The model under review builds one solid part; all positions refer to its coordinate system, in mm. A direction names the side the tool comes from. Round coordinates to 2 decimals unless told otherwise and drop trailing zeros. Order: outer loops, then holes, each group sorted by start corner. A loop starts at its lowest first (then second) coordinate and runs counter-clockwise, first axis right, second up. Notation, with made-up numbers: (-15, 65) -> (10, 65) arc R15 ccw to (10, 88) -> close; hole circle Ø3 at (56, -28). An arc over 180 degrees is marked (long way). Put each result on its own line as item: value. Start each with the question number.
from build123d import *

# Parameters (mm, degrees)
F1_DEPTH = 6
F2_DEPTH = 3
F3_START = 2
F3_DEPTH = 1
F4_SIZE  = 0.5
F5_DEPTH = 8
F6_START = -7.5
F6_DEPTH = 0.5
F7_R     = 0.49999


# Not quite as in the source:
# - a fillet or chamfer is up to 0.001 mm smaller than in the source, because OpenCascade refuses the exact size


with BuildPart() as f1:
    # F0 (on Front) → F1 (new body)
    with BuildSketch(Plane.XZ):
        with BuildLine():
            Line((2, 0), (4, 0))
            ThreePointArc((4, 0), (0, 4), (-4, 0))
            Line((-4, 0), (-2, 0))
            ThreePointArc((-2, 0), (-1.5491933385, 1.2649110641), (-0.4, 1.9595917942))
            Line((-0.4, 1.9595917942), (-0.4, 2))
            Line((-0.4, 2), (0, 2))
            Line((0, 2), (0.4, 2))
            Line((0.4, 2), (0.4, 1.9595917942))
            ThreePointArc((0.4, 1.9595917942), (1.5491933385, 1.2649110641), (2, 0))
        make_face()
        with BuildLine():
            Line((1.75, 0), (2, 0))
            ThreePointArc((2, 0), (1.5491933385, 1.2649110641), (0.4, 1.9595917942))
            Line((0.4, 1.9595917942), (0.4, 1.7036725037))
            ThreePointArc((0.4, 1.7036725037), (1.3715866724, 1.086853256), (1.75, 0))
        make_face()
        with BuildLine():
            ThreePointArc((-0.4, 1.9595917942), (-1.5491933385, 1.2649110641), (-2, 0))
            Line((-2, 0), (-1.75, 0))
            ThreePointArc((-1.75, 0), (-1.3715866724, 1.086853256), (-0.4, 1.7036725037))
            Line((-0.4, 1.7036725037), (-0.4, 1.9595917942))
        make_face()
        with BuildLine():
            Line((1.2, 0), (1.75, 0))
            ThreePointArc((1.75, 0), (1.3715866724, 1.086853256), (0.4, 1.7036725037))
            Line((0.4, 1.7036725037), (0.4, 1.1313708499))
            ThreePointArc((0.4, 1.1313708499), (0.9797958971, 0.692820323), (1.2, 0))
        make_face()
        with BuildLine():
            ThreePointArc((0, 2), (0.201017924, 1.989872306), (0.4, 1.9595917942))
            Line((0.4, 1.9595917942), (0.4, 2))
            Line((0.4, 2), (0, 2))
        make_face()
        with BuildLine():
            Line((0.4, 1.7036725037), (0.4, 1.9595917942))
            ThreePointArc((0.4, 1.9595917942), (0.201017924, 1.989872306), (0, 2))
            ThreePointArc((0, 2), (-0.201017924, 1.989872306), (-0.4, 1.9595917942))
            Line((-0.4, 1.9595917942), (-0.4, 1.7036725037))
            ThreePointArc((-0.4, 1.7036725037), (0, 1.75), (0.4, 1.7036725037))
        make_face()
        with BuildLine():
            ThreePointArc((-0.4, 1.7036725037), (-1.3715866724, 1.086853256), (-1.75, 0))
            Line((-1.75, 0), (-1.2, 0))
            ThreePointArc((-1.2, 0), (-0.9797958971, 0.692820323), (-0.4, 1.1313708499))
            Line((-0.4, 1.1313708499), (-0.4, 1.7036725037))
        make_face()
        with BuildLine():
            Line((-0.4, 2), (-0.4, 1.9595917942))
            ThreePointArc((-0.4, 1.9595917942), (-0.201017924, 1.989872306), (0, 2))
            Line((0, 2), (-0.4, 2))
        make_face()
        with BuildLine():
            Line((1, 0), (1.2, 0))
            ThreePointArc((1.2, 0), (0.9797958971, 0.692820323), (0.4, 1.1313708499))
            Line((0.4, 1.1313708499), (0.4, 0.916515139))
            ThreePointArc((0.4, 0.916515139), (0.8366600265, 0.5477225575), (1, 0))
        make_face()
        with BuildLine():
            Line((0.4, 1.1313708499), (0.4, 1.7036725037))
            ThreePointArc((0.4, 1.7036725037), (0, 1.75), (-0.4, 1.7036725037))
            Line((-0.4, 1.7036725037), (-0.4, 1.1313708499))
            ThreePointArc((-0.4, 1.1313708499), (0, 1.2), (0.4, 1.1313708499))
        make_face()
        with BuildLine():
            ThreePointArc((-0.4, 1.1313708499), (-0.9797958971, 0.692820323), (-1.2, 0))
            Line((-1.2, 0), (-1, 0))
            ThreePointArc((-1, 0), (-0.8366600265, 0.5477225575), (-0.4, 0.916515139))
            Line((-0.4, 0.916515139), (-0.4, 1.1313708499))
        make_face()
        with BuildLine():
            Line((0.4, 0), (1, 0))
            ThreePointArc((1, 0), (0.8366600265, 0.5477225575), (0.4, 0.916515139))
            Line((0.4, 0.916515139), (0.4, 0))
        make_face()
        with BuildLine():
            Line((0.4, 0.916515139), (0.4, 1.1313708499))
            ThreePointArc((0.4, 1.1313708499), (0, 1.2), (-0.4, 1.1313708499))
            Line((-0.4, 1.1313708499), (-0.4, 0.916515139))
            ThreePointArc((-0.4, 0.916515139), (0, 1), (0.4, 0.916515139))
        make_face()
        with BuildLine():
            ThreePointArc((-0.4, 0.916515139), (-0.8366600265, 0.5477225575), (-1, 0))
            Line((-1, 0), (-0.4, 0))
            Line((-0.4, 0), (-0.4, 0.916515139))
        make_face()
        with BuildLine():
            Line((-0.4, 0), (0.4, 0))
            Line((0.4, 0), (0.4, 0.916515139))
            ThreePointArc((0.4, 0.916515139), (0, 1), (-0.4, 0.916515139))
            Line((-0.4, 0.916515139), (-0.4, 0))
        make_face()
    extrude(amount=-F1_DEPTH)

    # F0 (on Front) → F2 (join)
    with BuildSketch(Plane.XZ):
        with BuildLine():
            ThreePointArc((-0.4, 1.7036725037), (-1.3715866724, 1.086853256), (-1.75, 0))
            Line((-1.75, 0), (-1.2, 0))
            ThreePointArc((-1.2, 0), (-0.9797958971, 0.692820323), (-0.4, 1.1313708499))
            Line((-0.4, 1.1313708499), (-0.4, 1.7036725037))
        make_face()
        with BuildLine():
            Line((1, 0), (1.2, 0))
            ThreePointArc((1.2, 0), (0.9797958971, 0.692820323), (0.4, 1.1313708499))
            Line((0.4, 1.1313708499), (0.4, 0.916515139))
            ThreePointArc((0.4, 0.916515139), (0.8366600265, 0.5477225575), (1, 0))
        make_face()
        with BuildLine():
            Line((1.2, 0), (1.75, 0))
            ThreePointArc((1.75, 0), (1.3715866724, 1.086853256), (0.4, 1.7036725037))
            Line((0.4, 1.7036725037), (0.4, 1.1313708499))
            ThreePointArc((0.4, 1.1313708499), (0.9797958971, 0.692820323), (1.2, 0))
        make_face()
        with BuildLine():
            ThreePointArc((-0.4, 1.1313708499), (-0.9797958971, 0.692820323), (-1.2, 0))
            Line((-1.2, 0), (-1, 0))
            ThreePointArc((-1, 0), (-0.8366600265, 0.5477225575), (-0.4, 0.916515139))
            Line((-0.4, 0.916515139), (-0.4, 1.1313708499))
        make_face()
    extrude(amount=F2_DEPTH)

    # F0 (on Front) → F3 (join)
    with BuildSketch(Plane.XZ.offset(F3_START)):
        with BuildLine():
            Line((1.75, 0), (2, 0))
            ThreePointArc((2, 0), (1.5491933385, 1.2649110641), (0.4, 1.9595917942))
            Line((0.4, 1.9595917942), (0.4, 1.7036725037))
            ThreePointArc((0.4, 1.7036725037), (1.3715866724, 1.086853256), (1.75, 0))
        make_face()
        with BuildLine():
            ThreePointArc((-0.4, 1.9595917942), (-1.5491933385, 1.2649110641), (-2, 0))
            Line((-2, 0), (-1.75, 0))
            ThreePointArc((-1.75, 0), (-1.3715866724, 1.086853256), (-0.4, 1.7036725037))
            Line((-0.4, 1.7036725037), (-0.4, 1.9595917942))
        make_face()
    extrude(amount=F3_DEPTH)

    # F4
    f4_edges = [f1.edges().sort_by_distance(p)[0] for p in [
        (0, 0, 4),
        (0, 6, 4),
    ]]
    chamfer(f4_edges, length=F4_SIZE)

    # F0 (on Front) → F5 (join)
    with BuildSketch(Plane.XZ):
        with BuildLine():
            Line((0.4, 0), (1, 0))
            ThreePointArc((1, 0), (0.8366600265, 0.5477225575), (0.4, 0.916515139))
            Line((0.4, 0.916515139), (0.4, 0))
        make_face()
        with BuildLine():
            ThreePointArc((-0.4, 0.916515139), (-0.8366600265, 0.5477225575), (-1, 0))
            Line((-1, 0), (-0.4, 0))
            Line((-0.4, 0), (-0.4, 0.916515139))
        make_face()
    extrude(amount=-F5_DEPTH)

    # F0 (on Front) → F6 (join)
    with BuildSketch(Plane.XZ.offset(F6_START)):
        with BuildLine():
            ThreePointArc((-0.4, 1.1313708499), (-0.9797958971, 0.692820323), (-1.2, 0))
            Line((-1.2, 0), (-1, 0))
            ThreePointArc((-1, 0), (-0.8366600265, 0.5477225575), (-0.4, 0.916515139))
            Line((-0.4, 0.916515139), (-0.4, 1.1313708499))
        make_face()
        with BuildLine():
            Line((1, 0), (1.2, 0))
            ThreePointArc((1.2, 0), (0.9797958971, 0.692820323), (0.4, 1.1313708499))
            Line((0.4, 1.1313708499), (0.4, 0.916515139))
            ThreePointArc((0.4, 0.916515139), (0.8366600265, 0.5477225575), (1, 0))
        make_face()
    extrude(amount=-F6_DEPTH)

    # F7 (radius 0.5 in the source; OpenCascade refuses exactly that, so slightly less here)
    f7_edges = [f1.edges().sort_by_distance(p)[0] for p in [
        (0.979796, 8, 0.69282),
        (-0.979796, 8, 0.69282),
        (1.549193, -3, 1.264911),
        (-1.549193, -3, 1.264911),
    ]]
    fillet(f7_edges, radius=F7_R)


solid = f1.part
Q1. Clearance check with flat-ended pins moving along their axes: pin 1 Ø2 at (x, z) = (-1, 1.5) entering from +Y; pin 2 Ø0.8 at (x, z) = (-1, 1) entering from +Y; pin 3 Ø0.5 at (x, z) = (1.5, 1) entering from +Y. State where each tip first meets the part, or that it passes through.
Q2. Take a section at B-B on y = 5. Give the boundary of the cut face in (x, z), and give its area (3 significant figures).
Q3. Take a section at A-A on x = 0. Give the boundary of the cut face in (y, z), and give its area (4 significant figures).
Q4. Wall thickness on probe 1 along Y at (x, z) = (3, 1.35); probe 2 along X at (y, z) = (4, 1.9); probe 3 along X at (y, z) = (-2.25, 1.3): over which ranges is each line inside the solid? List them lowest first. Write a range as [from, to].
Q5. Draft analysis for pull direction X (two halves, no side actions). For faces 5 (the face through (0.4, 7, 0.4)), 6 (the face through (0, 3, 4)), 7 (the face through (0.94, -3, 0.73)), state which applies: +X half, -X half, draft (parallel to the pull), parting line (faces both ways), or undercut.
Q6. For faces 1 (the face through (1.56, -2.25, 1.25)), 2 (the face through (1.382, -0.986, 1.074)), 3 (the face through (-1.537, -2.247, 1.28)), 4 (the face through (-0.4, -1.5, 1.3)), list the 3-axis set-ups (+Z, -Z, +X, -X, +Y, -Y) from which the entire face can be reached by the end or side of a thin tool; tool diameter is ignored.
Calculated:
1. pin 1: stops at y = 7.99
1. pin 2: stops at y = 7.89
1. pin 3: stops at y = 6
2. outline: (-4, 0) -> (4, 0) arc R4 ccw to start
2. area: 25.1 mm²
3. outline: (0, 0) -> (6, 0) -> (6, 3.5) -> (5.5, 4) -> (0.5, 4) -> (0, 3.5) -> close
3. area: 23.75 mm²
4. probe 1: y = [0, 6]
4. probe 2: x = [-3.52, 3.52]
4. probe 3: x = [-1.52, -0.4], [0.4, 1.52]
5. face 5: undercut
5. face 6: parting line
5. face 7: draft
6. face 1: +Z, +X, -Y
6. face 2: +Z, +X
6. face 3: +Z, -X, -Y
6. face 4: +Z, -Z, -Y
